Autodesk Inventor part; units mm, degrees
ref_plane "YZ Plane" through (0, 0, 0) normal (1, 0, 0) x (0, 1, 0)
ref_plane "XZ Plane" through (0, 0, 0) normal (0, 1, 0) x (-1, 0, 0)
ref_plane "XY Plane" through (0, 0, 0) normal (0, 0, 1) x (1, 0, 0)
sketch "Sketch1" plane through (0, 0, 0) normal (1, 0, 0) x (0, 1, 0)
  line L0 (7.5, 25) -> (-7.5, 25)
  line L1 (-7.5, 25) -> (-7.5, -25)
  line L2 (-7.5, -25) -> (7.5, -25)
  line L3 (7.5, -25) -> (7.5, 25)
  point P0 (0, 0)
  dimension "d0" = 50
  dimension "d1" = 25
  dimension "d2" = 15
  dimension "d3" = 7.5
extrude "Extrusion1" add sketch "Sketch1" against normal blind 5
sketch "Sketch2" plane through (0, 0, 0) normal (1, 0, 0) x (0, 0, -1)
  circle A0 centre (-12.1, 4) radius 0.55
  circle A1 centre (-14.95, 4) radius 1
  circle A2 centre (4.25, 4) radius 0.55
  circle A3 centre (7.1, 4) radius 1
  line L0 (25, -7.5) -> (25, 7.5)
  line L1 (-25, 7.5) -> (-25, -7.5)
  line L2 (-14.95, 4) -> (7.1, 4) construction
  line L3 (-25, -7.5) -> (25, -7.5)
  point P0 (0, 0)
  dimension "d6" = 2
  dimension "d7" = 2
  dimension "d8" = 1.1
  dimension "d9" = 1.1
  dimension "d11" = 2.85
  dimension "d13" = 2.85
  dimension "d14" = 10.05
  dimension "d15" = 11.5
  dimension "d19" = 16.35
extrude "Extrusion2" cut sketch "Sketch2" against normal up to surface (5 mm away)
fillet "Fillet1" radius 0.5 8 edges at (0, 0, 25) (0, 7.5, 0) (0, 0, -25) (0, -7.5, 0) (-2.5, 7.5, 25) (-2.5, -7.5, 25) (-2.5, 7.5, -25) (-2.5, -7.5, -25)
properties part number "Backplate"
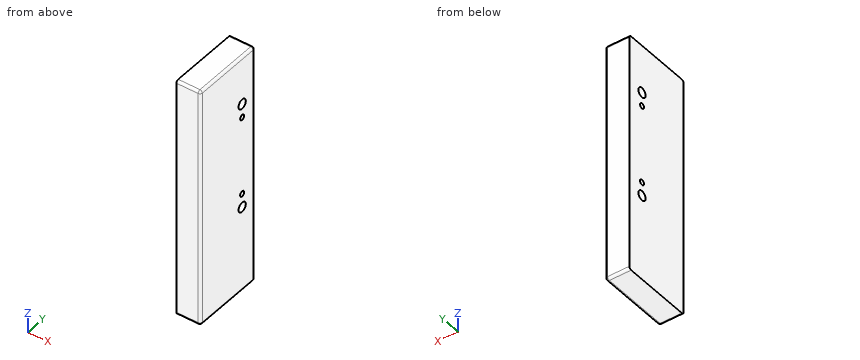
Geometry: final body of the model. Coordinates: model frame, mm. Give positions to 0.01 mm unless a question says otherwise; leave off trailing zeros. Write each loop counter-clockwise with the first axis right and the second up, starting at its lowest first coordinate (ties: lowest second). Pieces come first, ordered by that corner, then holes. Notation, with made-up numbers: M -9.5,38.5 L 2.5,38.5 A20 cw 2.5,47.5 Z; hole C -32,-0.75 d7. An arc over 180 degrees is marked long. Answer in a Markdown table with one row per item. Add a question column.
(1) Section B-B on y = 4. Return loops of the section in (x, z), and give its area (3 significant figures).
(2) Section A-A on z = -7.1. Return loops of the section in (x, y), and give its area (3 significant figures).
(3) Section C-C on z = 14.5. Return loops of the section in (x, y).
(4) Ray query, line 1 (Y direction, x = -1.7, z = -7.1); line 2 (Y direction, x = -1.65, z = 12.1); line 3 (Z direction, x = -2.8, y = 4.25). Return the intervals inside material, ascending.
Result set:
| question | item | result |
|---|---|---|
| 1 | outline | M -5,-25 L -0.5,-25 A0.5 ccw 0,-24.5 L 0,-8.1 L -5,-8.1 Z; M -5,-6.1 L 0,-6.1 L 0,-4.8 L -5,-4.8 Z; M -5,-3.7 L 0,-3.7 L 0,11.55 L -5,11.55 Z; M -5,12.65 L 0,12.65 L 0,13.95 L -5,13.95 Z; M -5,15.95 L 0,15.95 L 0,24.5 A0.5 ccw -0.5,25 L -5,25 Z |
| 1 | area | 219 mm^2 |
| 2 | outline | M -5,-7.5 L -0.5,-7.5 A0.5 ccw 0,-7 L 0,3 L -5,3 Z; M -5,5 L 0,5 L 0,7 A0.5 ccw -0.5,7.5 L -5,7.5 Z |
| 2 | area | 64.9 mm^2 |
| 3 | outline | M -5,-7.5 L -0.5,-7.5 A0.5 ccw 0,-7 L 0,3.11 L -5,3.11 Z; M -5,4.89 L 0,4.89 L 0,7 A0.5 ccw -0.5,7.5 L -5,7.5 Z |
| 4 | line 1 | y = -7.5 to 3, 5 to 7.5 |
| 4 | line 2 | y = -7.5 to 3.45, 4.55 to 7.5 |
| 4 | line 3 | z = -25 to -8.07, -6.13 to -4.74, -3.76 to 11.61, 12.59 to 13.98, 15.92 to 25 |
